from build123d import *

# Parameters (mm, degrees)
F0_R      = 7
F1_DEPTH  = 28.8
F4_DEPTH  = 12
F6_DEPTH  = 10
F8_DEPTH  = 10
F9_R      = 3.4
F10_DEPTH = 12
F11_R     = 2
F12_R     = 4


with BuildPart() as f1:
    # F0 (on Right) → F1 (new body)
    with BuildSketch(Plane.YZ):
        with BuildLine():
            Line((120, 0), (12, 0))
            ThreePointArc((12, 0), (-8.4852813742, 8.4852813742), (0, -12))
            Line((0, -12), (120, -12))
            Line((120, -12), (120, 0))
        make_face()
        Circle(F0_R, mode=Mode.SUBTRACT)
    extrude(amount=F1_DEPTH)

    # F3 (on offset) → F4 (cut)
    with BuildSketch(Plane.YZ.offset(20.4)):
        with BuildLine():
            Line((14, -12), (14, 0))
            Line((14, 0), (12, 0))
            ThreePointArc((12, 0), (-8.4852813742, 8.4852813742), (0, -12))
            Line((0, -12), (14, -12))
        make_face()
    extrude(amount=-F4_DEPTH, mode=Mode.SUBTRACT)

    # F5 (on face) → F6 (join)
    with BuildSketch(Plane.YZ.offset(28.8)):
        with BuildLine():
            Line((65, 0), (75, 0))
            Line((75, 0), (75, 20))
            Line((75, 20), (65, 20))
            ThreePointArc((65, 20), (63.0248532563, 9.2952660561), (57.36, 0))
            Line((57.36, 0), (65, 0))
        make_face()
    extrude(amount=-F6_DEPTH)

    # F7 (on face) → F8 (cut, through all)
    with BuildSketch(Plane.YZ.offset(28.8)):
        Polygon((57.36, -12), (57.36, 0), (42.36, 0), (47.36, -12), align=None)
    extrude(amount=-F8_DEPTH, mode=Mode.SUBTRACT)

    # F9 (on Top) → F10 (cut, through all)
    with BuildSketch(Plane.XY):
        with Locations((9.4, 97)):
            Circle(F9_R)
    extrude(amount=-F10_DEPTH, mode=Mode.SUBTRACT)

    # F11
    f11_edges = [f1.edges().sort_by_distance(p)[0] for p in [
        (23.8, 75, 0),
        (24.6, 12, 0),
        (4.2, 12, 0),
    ]]
    fillet(f11_edges, radius=F11_R)

    # F12
    f12_edges = [f1.edges().sort_by_distance(p)[0] for p in [
        (23.8, 75, 20),
        (14.4, 120, 0),
    ]]
    fillet(f12_edges, radius=F12_R)


solid = f1.part
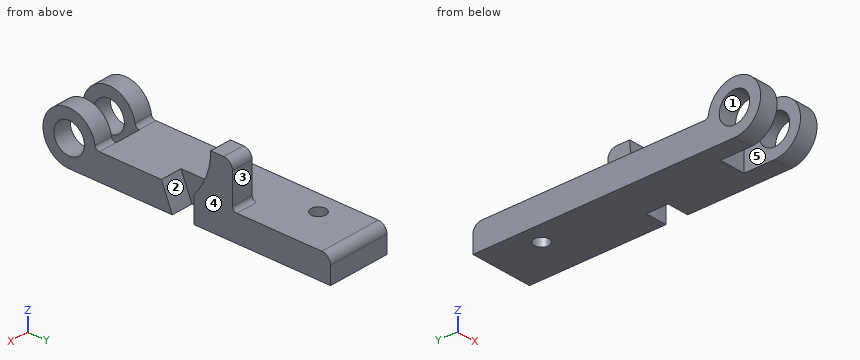
Geometry: final body of the model. Coordinates: model frame, mm. Face numbers are marked on the shaded views. A direction names the side the tool comes from. Coordinates: 2 decimals unless noted, no trailing zeros. Order: outer loops, then holes, each group sorted by start corner. A loop starts at its lowest first (then second) coordinate and runs counter-clockwise, first axis right, second up.
1) Draft query along X for the marked faces 3, 4 and 5. Return one class per face: released by +X, released by -X, zero draft, split by the parting line, or undercut.
Result sheet:
face 3: zero draft
face 4: released by +X
face 5: undercut
2) Section B-B (x = 4). Return loops of the section in (y, z).
Result sheet:
outline: (0, -12) - (120, -12) - (120, -4) arc R4 ccw to (116, 0) - (13.86, 0) arc R2 cw to (11.88, 1.71) arc R12 ccw (long way) to start; hole circle Ø14 at (0, 0)
3) First-contact query: P1, Ø12, axis at y = 75.5, z = 0, coming from the -X side; P2, Ø8, axis at x = 17.5, z = 11.5, coming from the +Y side; P3, Ø6, axis at y = 71, z = 5.5, coming from the -X side; P4, Ø8, axis at x = 24, z = -5.5, coming from the -Y side. Flat tips, straight axial feed; report the tip coordinate or a pass-through.
Result sheet:
P1: stops at x = 0
P2: stops at y = 75
P3: stops at x = 18.8
P4: stops at y = -11.91
4) Ray query, probe 1 along Z at (x, y) = (23.75, 0); probe 2 along Y at (x, z) = (9.4, -4.5); probe 3 along Z at (x, y) = (9.5, 108). Return the intervals inside material, ascending.
Result sheet:
probe 1: z = -12 to -7, 7 to 12
probe 2: y = 14 to 93.6, 100.4 to 120
probe 3: z = -12 to 0
5) Section A-A (y = 97). Return loops of the section in (x, z).
Result sheet:
outline: (0, -12) - (6, -12) - (6, 0) - (0, 0) - close; (12.8, -12) - (28.8, -12) - (28.8, 0) - (12.8, 0) - close
6) Section C-C (x = 10.25). Return loops of the section in (y, z).
Result sheet:
outline: (14, -12) - (93.71, -12) - (93.71, 0) - (14, 0) - close; (100.29, -12) - (120, -12) - (120, -4) arc R4 ccw to (116, 0) - (100.29, 0) - close
7) Set-up query: the marked faces 1 and 2. Return all of +Z, -Z, +X, -X, +Y, -Y with unobstructed straight access to the full face (end or side cutting, diameter ignored); none if empty.
Result sheet:
face 1: +X, -X
face 2: +Z, +X
8) Section D-D (y = -2). Return loops of the section in (x, z).
Result sheet:
outline: (0, -11.83) - (8.4, -11.83) - (8.4, -6.71) - (0, -6.71) - close; (0, 6.71) - (8.4, 6.71) - (8.4, 11.83) - (0, 11.83) - close; (20.4, -11.83) - (28.8, -11.83) - (28.8, -6.71) - (20.4, -6.71) - close; (20.4, 6.71) - (28.8, 6.71) - (28.8, 11.83) - (20.4, 11.83) - close
